Geometry check sheet. Reference: the model listing, model coordinates, mm. Face numbers are marked on the shaded views. A direction names the side the tool comes from. Give positions to 0.01 mm unless a question says otherwise; leave off trailing zeros. Order: outer loops, then holes, each group sorted by start corner. A loop starts at its lowest first (then second) coordinate and runs counter-clockwise, first axis right, second up.
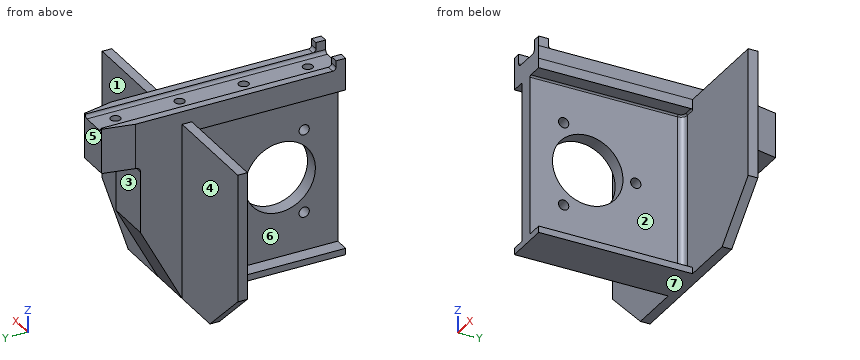
from build123d import *

# Parameters (mm, degrees)
EXTRUDE_2_DEPTH      = 55
SKETCH_5_W           = 50
SKETCH_5_H           = 58
CUT_EXTRUDE_2_DEPTH  = 4.5
SKETCH_6_R           = 11
SKETCH_6_R_2         = 1.6
CUT_EXTRUDE_3_DEPTH  = 4.5
SKETCH_8_W           = 14.000064841
SKETCH_8_H           = 24
EXTRUDE_3_DEPTH      = 55
SKETCH_9_R           = 1.55
CUT_EXTRUDE_4_DEPTH  = 4
CUT_EXTRUDE_8_DEPTH  = 55
CUT_EXTRUDE_12_DEPTH = 15
CUT_EXTRUDE_13_DEPTH = 3
SKETCH_23_W          = 50
SKETCH_23_H          = 58
CUT_EXTRUDE_14_DEPTH = 5
SKETCH_24_W          = 14
SKETCH_24_H          = 10
CUT_EXTRUDE_15_DEPTH = 56
FILLET_1_R           = 2
FILLET_2_R           = 2
FILLET_3_R           = 0.5
CUT_EXTRUDE_16_DEPTH = 11
FILLET_4_R           = 1.5
EXTRUDE_START        = 4
SKETCH_26_R          = 1.55
EXTRUDE_4_DEPTH      = 4
SKETCH_27_W          = 9
SKETCH_27_H          = 75
CUT_EXTRUDE_17_DEPTH = 1
FILLET_5_R           = 1
SKETCH_28_W          = 2.500032421
SKETCH_28_H          = 3
SKETCH_28_W_2        = 2.499970549
EXTRUDE_5_DEPTH      = 3
FILLET_6_R           = 1
SKETCH_29_R          = 1.55
CUT_EXTRUDE_18_DEPTH = 11


# Some blends are built 0.0001 mm under size
with BuildPart() as part:
    # 草图4 → 凸台-拉伸2 (new body)
    with BuildSketch(Plane.XY):
        Polygon((-14.679245283, 23.924528302), (63.320754717, 23.924528302), (63.320754717, 20.924528302), (31.320754717, 20.924528302), (31.320754717, -37.075471698), (17.320754717, -37.075471698), (17.320754717, 20.924528302), (-14.679245283, 20.924528302), align=None)
    extrude(amount=EXTRUDE_2_DEPTH)

    # 草图5 → 切除-拉伸2 (cut)
    with BuildSketch(Plane.ZY.offset(-17.320754717)):
        with Locations((27, -8.075471698)):
            Rectangle(SKETCH_5_W, SKETCH_5_H)
    extrude(amount=-CUT_EXTRUDE_2_DEPTH, mode=Mode.SUBTRACT)

    # 草图6 → 切除-拉伸3 (cut)
    with BuildSketch(Plane.ZY.offset(-21.820754717)):
        with Locations((27, -9.075471698)):
            Circle(SKETCH_6_R)
        with Locations((27, 5.924528302)):
            Circle(SKETCH_6_R_2)
        with Locations((39.990381057, -16.575471698)):
            Circle(SKETCH_6_R_2)
        with Locations((14.009618943, -16.575471698)):
            Circle(SKETCH_6_R_2)
    extrude(amount=-CUT_EXTRUDE_3_DEPTH, mode=Mode.SUBTRACT)

    # 草图8 → 凸台-拉伸3 (add)
    with BuildSketch(Plane.XY.offset(55)):
        with Locations((24.320787138, 35.924528302)):
            Rectangle(SKETCH_8_W, SKETCH_8_H)
    extrude(amount=-EXTRUDE_3_DEPTH)

    # 草图9 → 切除-拉伸4 (cut)
    with BuildSketch(Plane.XY.offset(55)):
        with Locations((24.320784468, 40.924528302)):
            Circle(SKETCH_9_R)
        with Locations((24.320784468, 20.924528302)):
            Circle(SKETCH_9_R)
        with Locations((24.320784468, 0.924528302)):
            Circle(SKETCH_9_R)
        with Locations((24.320784468, -19.075471698)):
            Circle(SKETCH_9_R)
    extrude(amount=-CUT_EXTRUDE_4_DEPTH, mode=Mode.SUBTRACT)

    # 草图13 → 切除-拉伸8 (cut)
    with BuildSketch(Plane.XY.offset(55)):
        Polygon((17.320754717, 47.924528302), (19.320754717, 47.924528302), (17.320754717, 38.424528302), align=None)
        Polygon((29.320819558, 47.924528302), (31.320819558, 47.924528302), (31.320819558, 38.424528302), align=None)
    extrude(amount=-CUT_EXTRUDE_8_DEPTH, mode=Mode.SUBTRACT)

    # 草图20 → 切除-拉伸12 (cut)
    with BuildSketch(Plane(origin=(31.320819558, 0, 0), x_dir=(0, 0, -1), z_dir=(1, 0, 0))):
        Polygon((0, 23.924528302), (0, 47.924528302), (-45, 47.924528302), align=None)
    extrude(amount=-CUT_EXTRUDE_12_DEPTH, mode=Mode.SUBTRACT)

    # 草图21 → 切除-拉伸13 (cut)
    with BuildSketch(Plane(origin=(0, 23.924528302, 0), x_dir=(1, 0, 0), z_dir=(0, 1, 0))):
        Polygon((-14.679245283, 0), (1.320754717, 0), (-14.679245283, -15), align=None)
        Polygon((48.320754717, 0), (63.320754717, 0), (63.320754717, -15), align=None)
    extrude(amount=-CUT_EXTRUDE_13_DEPTH, mode=Mode.SUBTRACT)

    # 草图23 → 切除-拉伸14 (cut)
    with BuildSketch(Plane(origin=(31.320754717, 0, 0), x_dir=(0, 0, -1), z_dir=(1, 0, 0))):
        with Locations((-27, -8.075471698)):
            Rectangle(SKETCH_23_W, SKETCH_23_H)
    extrude(amount=-CUT_EXTRUDE_14_DEPTH, mode=Mode.SUBTRACT)

    # 草图24 → 切除-拉伸15 (cut)
    with BuildSketch(Plane.XY.offset(55)):
        with Locations((24.320754717, -32.075471698)):
            Rectangle(SKETCH_24_W, SKETCH_24_H)
    extrude(amount=-CUT_EXTRUDE_15_DEPTH, mode=Mode.SUBTRACT)

    # 圆角1
    fillet_1_edges = [part.edges().sort_by_distance(p)[0] for p in [
        (21.820754717, 20.924528302, 27),
    ]]
    fillet(fillet_1_edges, radius=FILLET_1_R)

    # 圆角2
    fillet_2_edges = [part.edges().sort_by_distance(p)[0] for p in [
        (26.320754717, 20.924528302, 27),
    ]]
    fillet(fillet_2_edges, radius=FILLET_2_R)

    # 圆角3
    fillet_3_edges = [part.edges().sort_by_distance(p)[0] for p in [
        (21.820754717, -4.075471698, 52),
        (18.570754717, 20.924528302, 52),
        (21.234968279, 20.338741864, 52),
        (26.320754717, -4.075471698, 52),
        (29.820754717, 20.924528302, 52),
        (26.906541155, 20.338741864, 52),
    ]]
    fillet(fillet_3_edges, radius=FILLET_3_R)

    # 草图25 → 切除-拉伸16 (cut)
    with BuildSketch(Plane(origin=(0, 47.924528302, 0), x_dir=(1, 0, 0), z_dir=(0, 1, 0))):
        Polygon((19.320754717, -45), (17.320754717, -45), (17.320754717, -24), (31.320819558, -24), (31.320819558, -45), align=None)
    extrude(amount=-CUT_EXTRUDE_16_DEPTH, mode=Mode.SUBTRACT)

    # 圆角4
    fillet_4_edges = [part.edges().sort_by_distance(p)[0] for p in [
        (24.320787138, 36.924528302, 45),
    ]]
    fillet(fillet_4_edges, radius=FILLET_4_R)

    # 草图26 → 凸台-拉伸4 (add)
    with BuildSketch(Plane.XY.offset(55).offset(EXTRUDE_START)):
        Polygon((17.320754717, -27.075471698), (31.320754717, -27.075471698), (31.320819558, 38.424528302), (29.320819558, 47.924528302), (19.320754717, 47.924528302), (17.320754717, 38.424528302), align=None)
        with Locations((24.320784468, -19.075471698)):
            Circle(SKETCH_26_R, mode=Mode.SUBTRACT)
        with Locations((24.320784468, 0.924528302)):
            Circle(SKETCH_26_R, mode=Mode.SUBTRACT)
        with Locations((24.320784468, 20.924528302)):
            Circle(SKETCH_26_R, mode=Mode.SUBTRACT)
        with Locations((24.320784468, 40.924528302)):
            Circle(SKETCH_26_R, mode=Mode.SUBTRACT)
    extrude(amount=-EXTRUDE_4_DEPTH)

    # 草图27 → 切除-拉伸17 (cut)
    with BuildSketch(Plane.XY.offset(59)):
        with Locations((24.320787138, 10.424528302)):
            Rectangle(SKETCH_27_W, SKETCH_27_H)
    extrude(amount=-CUT_EXTRUDE_17_DEPTH, mode=Mode.SUBTRACT)

    # 圆角5
    fillet_5_edges = [part.edges().sort_by_distance(p)[0] for p in [
        (28.820787138, 10.424528302, 58),
        (19.820787138, 10.424528302, 58),
    ]]
    fillet(fillet_5_edges, radius=FILLET_5_R - 0.0001)  # a hair under: the kernel refuses the full size

    # 草图28 → 凸台-拉伸5 (add)
    with BuildSketch(Plane.XY.offset(59)):
        with Locations((18.570770927, -25.575471698)):
            Rectangle(SKETCH_28_W, SKETCH_28_H)
        with Locations((30.070772412, -25.575471698)):
            Rectangle(SKETCH_28_W_2, SKETCH_28_H)
    extrude(amount=EXTRUDE_5_DEPTH)

    # 圆角6
    # the kernel refuses this fillet: 1 mm, written as the material it adds along each edge
    with BuildSketch(Plane(origin=(19.820787138, -24.075471698, 59), x_dir=(0, 0, 1), z_dir=(-1, 0, 0))) as fillet_6_piece_1:
        with BuildLine():
            CenterArc((FILLET_6_R, FILLET_6_R), FILLET_6_R, 180, 90)
            Line((0, FILLET_6_R), (0, 0))
            Line((0, 0), (FILLET_6_R, 0))
        make_face()
    extrude(amount=2.500032421)
    with BuildSketch(Plane(origin=(33.820757687, -24.075471698, 59), x_dir=(0, 1, 0), z_dir=(-1, 0, 0))) as fillet_6_piece_2_section:
        with BuildLine():
            CenterArc((FILLET_6_R, -FILLET_6_R), FILLET_6_R, 90, 90)
            Line((0, -FILLET_6_R), (0, 0))
            Line((0, 0), (FILLET_6_R, 0))
        make_face()
    fillet_6_piece_2 = extrude(amount=4.999970549, mode=Mode.PRIVATE)
    fillet_6_piece_2 = split(fillet_6_piece_2, bisect_by=Plane(origin=(31.320757908, -23.852105032, 59.223367959), z_dir=(-0.9999999999995101, 9.899447945822129e-07, 0)), keep=Keep.TOP, mode=Mode.PRIVATE)
    add(fillet_6_piece_2)

    # 草图29 → 切除-拉伸18 (cut)
    with BuildSketch(Plane.XY.offset(51)):
        with Locations((24.320784468, 40.924528302)):
            Circle(SKETCH_29_R)
    extrude(amount=-CUT_EXTRUDE_18_DEPTH, mode=Mode.SUBTRACT)


solid = part.part
Item 1: Draft check along Z on the marked faces 5, 6 and 7. Enter one of: released by +Z, released by -Z, zero draft, split by the parting line, or undercut.
Reported:
face 5: zero draft
face 6: undercut
face 7: released by -Z
Item 2: Gauge pin test, flat ends, axial feed: pin 1 (4 mm diameter, centred on y = 2, z = 9.5, fed in from -X); pin 2 (4 mm diameter, centred on y = -12.5, z = 13, fed in from +X); pin 3 (3.5 mm diameter, centred on y = 27, z = 60.5, fed in from +X); pin 4 (5 mm diameter, centred on x = 24.32, y = 0.92, fed in from -Z). Record the tip position at first contact, or that the pin passes through.
Reported:
pin 1: stops at x = 21.82
pin 2: stops at x = 26.32
pin 3: stops at x = 31.32
pin 4: stops at z = 0
Item 3: Sectioned sample at A-A (z = 27). Enter the section's corners in (x, y).
Reported:
outline: (-14.68, 20.92) - (19.82, 20.92) arc R2 cw to (21.82, 18.92) - (21.82, 7.52) - (26.32, 7.52) - (26.32, 18.92) arc R2 cw to (28.32, 20.92) - (63.32, 20.92) - (63.32, 23.92) - (31.32, 23.92) - (31.32, 36.92) - (17.32, 36.92) - (17.32, 23.92) - (-14.68, 23.92) - close; (21.82, -27.08) - (26.32, -27.08) - (26.32, -20.08) - (21.82, -20.08) - close; (21.82, 1.92) - (26.32, 1.92) - (26.32, 4.32) - (21.82, 4.32) - close
Item 4: Scan lines: L1, parallel to Y at x = 23, z = 27; L2, parallel to Y at x = 41.5, z = 50.5; L3, parallel to Z at x = 30, y = -21.5. Record each from-to range of solid material in increasing order.
Reported:
L1: y = -27.08 to -20.08, 1.92 to 4.32, 7.52 to 36.92
L2: y = 20.92 to 23.92
L3: z = 0 to 2, 52 to 59
Item 5: Sectioned sample at D-D (z = 7). Enter the section's corners in (x, y).
Reported:
outline: (-6.15, 20.92) - (19.82, 20.92) arc R2 cw to (21.82, 18.92) - (21.82, -27.08) - (26.32, -27.08) - (26.32, 18.92) arc R2 cw to (28.32, 20.92) - (55.32, 20.92) - (55.32, 23.92) - (31.32, 23.92) - (31.32, 27.66) - (17.32, 27.66) - (17.32, 23.92) - (-6.15, 23.92) - close
Item 6: Set-up check for the marked faces 1, 2, 3 and 4: record each of +Z, -Z, +X, -X, +Y, -Y from which the full face is reachable in a straight line by a thin tool's end or side.
Reported:
face 1: +Z, -Z, +X, +Y
face 2: +X, -Y
face 3: -Z, +X, -X, +Y
face 4: +Z, -Z, -X, +Y
